Check sheet for the modelled part. Datum: model origin and axes. Units: mm. Round coordinates to 2 decimals unless told otherwise and drop trailing zeros. Order: outer loops, then holes, each group sorted by start corner. A loop starts at its lowest first (then second) coordinate and runs counter-clockwise, first axis right, second up.
Q1. Cross-section at A-A on z = 0.5. Record the cut outline in (x, y), then the cut area to 3 significant figures.
Q2. Depth check by flat-ended pin: P1, Ø3, axis at y = 9, z = 1, coming from the -X side. Enter the tip coordinate at first touch or a pass-through.
Q3. Scan line: probe 1 along Y at (x, z) = (137, -10.5). Record every from-to range of solid material in increasing order.
Q4. Cross-section at C-C on x = -498. Record the cut outline in (y, z).
from build123d import *

# Parameters (mm, degrees)
SKETCH2_W                = 25.54
SKETCH2_H                = 25.54
SKETCH2_W_2              = 22.365
SKETCH2_H_2              = 22.365
BOSS_EXTRUDE1_DEPTH      = 400
BOSS_EXTRUDE1_DEPTH_BACK = 590
FILLET1_R                = 1


with BuildPart() as part:
    # Sketch2 → Boss-Extrude1 (new body, two sides)
    with BuildSketch(Plane(origin=(0, 0, 0), x_dir=(0, 0, -1), z_dir=(1, 0, 0))) as boss_extrude1_sk:
        Rectangle(SKETCH2_W, SKETCH2_H)
        Rectangle(SKETCH2_W_2, SKETCH2_H_2, mode=Mode.SUBTRACT)
    extrude(amount=BOSS_EXTRUDE1_DEPTH)
    extrude(boss_extrude1_sk.sketch, amount=-BOSS_EXTRUDE1_DEPTH_BACK)

    # Fillet1
    fillet1_edges = [part.edges().sort_by_distance(p)[0] for p in [
        (-95, -12.77, -12.77),
        (-95, -12.77, 12.77),
        (-95, 12.77, 12.77),
        (-95, 12.77, -12.77),
    ]]
    fillet(fillet1_edges, radius=FILLET1_R)


solid = part.part
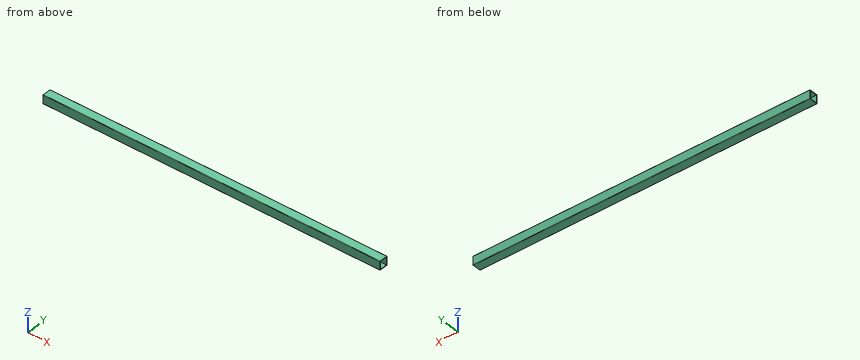
Results found:
1. outline: (-590, -12.77) - (400, -12.77) - (400, -11.18) - (-590, -11.18) - close; (-590, 11.18) - (400, 11.18) - (400, 12.77) - (-590, 12.77) - close
1. area: 3,140 mm2
2. P1: passes through
3. probe 1: y = -12.77 to -11.18, 11.18 to 12.77
4. outline: (-12.77, -11.77) arc R1 ccw to (-11.77, -12.77) - (11.77, -12.77) arc R1 ccw to (12.77, -11.77) - (12.77, 11.77) arc R1 ccw to (11.77, 12.77) - (-11.77, 12.77) arc R1 ccw to (-12.77, 11.77) - close; hole (-11.18, -11.18) - (11.18, -11.18) - (11.18, 11.18) - (-11.18, 11.18) - close
